```python
from build123d import *

# Parameters (mm, degrees)
SKETCH1_W           = 10
SKETCH1_H           = 10
BOSS_EXTRUDE1_DEPTH = 50
SKETCH3_W           = 10
SKETCH3_H           = 10
BOSS_EXTRUDE3_DEPTH = 11
SKETCH8_W           = 20
SKETCH8_H           = 10
BOSS_EXTRUDE4_DEPTH = 23
SKETCH9_R           = 2
CUT_EXTRUDE2_DEPTH  = 23
SKETCH9_4_R         = 2
CUT_EXTRUDE3_DEPTH  = 23


with BuildPart() as part:
    # Sketch1 → Boss-Extrude1 (new body)
    with BuildSketch(Plane.XY):
        with Locations((-2.851282988, -1.356707317)):
            Rectangle(SKETCH1_W, SKETCH1_H)
    extrude(amount=BOSS_EXTRUDE1_DEPTH)

    # Sketch3 → Boss-Extrude3 (add)
    with BuildSketch(Plane.ZY.offset(7.851282988)):
        with Locations((45, -1.356707317)):
            Rectangle(SKETCH3_W, SKETCH3_H)
    extrude(amount=BOSS_EXTRUDE3_DEPTH)

    # Sketch8 → Boss-Extrude4 (add)
    with BuildSketch(Plane(origin=(0, 3.643292683, 0), x_dir=(1, 0, 0), z_dir=(0, 1, 0))):
        with Locations((-8.851282988, -45)):
            Rectangle(SKETCH8_W, SKETCH8_H)
    extrude(amount=BOSS_EXTRUDE4_DEPTH)

    # Sketch9 → Cut-Extrude2 (cut)
    with BuildSketch(Plane(origin=(0, 3.643292683, 0), x_dir=(1, 0, 0), z_dir=(0, 1, 0))):
        with Locations(Location((-2.851282988, -7, 0), (0, 0, 270))):
            Circle(SKETCH9_R)
    extrude(amount=-CUT_EXTRUDE2_DEPTH, mode=Mode.SUBTRACT)

    # Sketch9_4 → Cut-Extrude3 (cut)
    with BuildSketch(Plane(origin=(0, 3.643292683, 0), x_dir=(1, 0, 0), z_dir=(0, 1, 0))):
        with Locations(Location((-2.851282988, -26, 0), (0, 0, 270))):
            Circle(SKETCH9_4_R)
    extrude(amount=-CUT_EXTRUDE3_DEPTH, mode=Mode.SUBTRACT)


solid = part.part
```
Model file for the job. Use its own axes, mm. A direction names the side the tool comes from. Give positions to 0.01 mm unless a question says otherwise; leave off trailing zeros. Write each loop counter-clockwise with the first axis right and the second up, starting at its lowest first coordinate (ties: lowest second). Pieces come first, ordered by that corner, then holes. Notation, with made-up numbers: (-33, 72.25) - (4, 72.25) arc R28 ccw to (4, 104.25) - close; hole circle Ø8 at (-3.5, 27). An arc over 180 degrees is marked (long way). One line per question, with ' | ' between items. Start each with the question number.
(1) Slice it at C-C on z = 6.5. Write the cut outline in (x, y), plus the area to 3 significant figures.
(2) 3-axis set-ups, long thin cutter, end or side, ignore diameter. For faces 4 (the face through (-9, 14, 40)), 5 (the face through (1.149, 15, 45)), 6 (the face through (-3, -1, 0)), 7 (the face through (-7.851, -1, 20)): which of +Z, -Z, +X, -X, +Y, -Y reach the whole face in a straight line?
(3) Slice it at A-A on z = 25. Write the cut outline in (x, y), plus the area to 3 significant figures.
(4) Slice it at D-D on x = -9.75. Write the cut outline in (y, z).
(5) Wall check: line 1 along Z through (x, y) = (-3, -1); line 2 along X through (y, z) = (-0.5, 26); line 3 along Z through (x, y) = (-13.25, 0). Give the ranges that are in metal, low to high. Write a range as from..to.
(6) Slice it at B-B on y = 3. Write the cut outline in (x, z), plus the area to 3 significant figures.
(7) Pin check, flat tips, straight feed: P1, Ø11, axis at y = 0.5, z = 25.5, coming from the -X side; P2, Ø5, axis at x = -5, z = 34, coming from the +Y side; P3, Ø8, axis at y = 15.5, z = 46.5, coming from the +X side. Stop position of each tip, or through.
(8) Two-plate mould, pull along Z, no slides. Class faces 1 (the face through (-9, 26.643, 45)), 2 (the face through (-2.251, -1.287, 27.908)), 3 (the face through (-8, 10, 50)): +Z half, -Z half, draft (parallel to the pull), parting line (faces both ways), or undercut.
Results below:
1) outline: (-7.85, -6.36) - (-4.79, -6.36) - (-4.79, 3.64) - (-7.85, 3.64) - close; (-0.91, -6.36) - (2.15, -6.36) - (2.15, 3.64) - (-0.91, 3.64) - close | area: 61.3 mm^2
2) face 4: -Z, -X, +Y | face 5: +Z, -Z, +X, +Y | face 6: -Z, +X, -X, +Y, -Y | face 7: -Z, -X, +Y, -Y
3) outline: (-7.85, -6.36) - (-4.58, -6.36) - (-4.58, 3.64) - (-7.85, 3.64) - close; (-1.12, -6.36) - (2.15, -6.36) - (2.15, 3.64) - (-1.12, 3.64) - close | area: 65.4 mm^2
4) outline: (-6.36, 40) - (26.64, 40) - (26.64, 50) - (-6.36, 50) - close
5) line 1: 0..5.01, 8.99..24.01, 27.99..50 | line 2: -7.85..-4.85, -0.85..2.15 | line 3: 40..50
6) outline: (-18.85, 40) - (-7.85, 40) - (-7.85, 0) - (2.15, 0) - (2.15, 50) - (-18.85, 50) - close; hole circle Ø4 at (-2.85, 7); hole circle Ø4 at (-2.85, 26) | area: 585 mm^2
7) P1: x = -7.85 | P2: y = 3.64 | P3: x = 1.15
8) face 1: draft | face 2: undercut | face 3: +Z half
